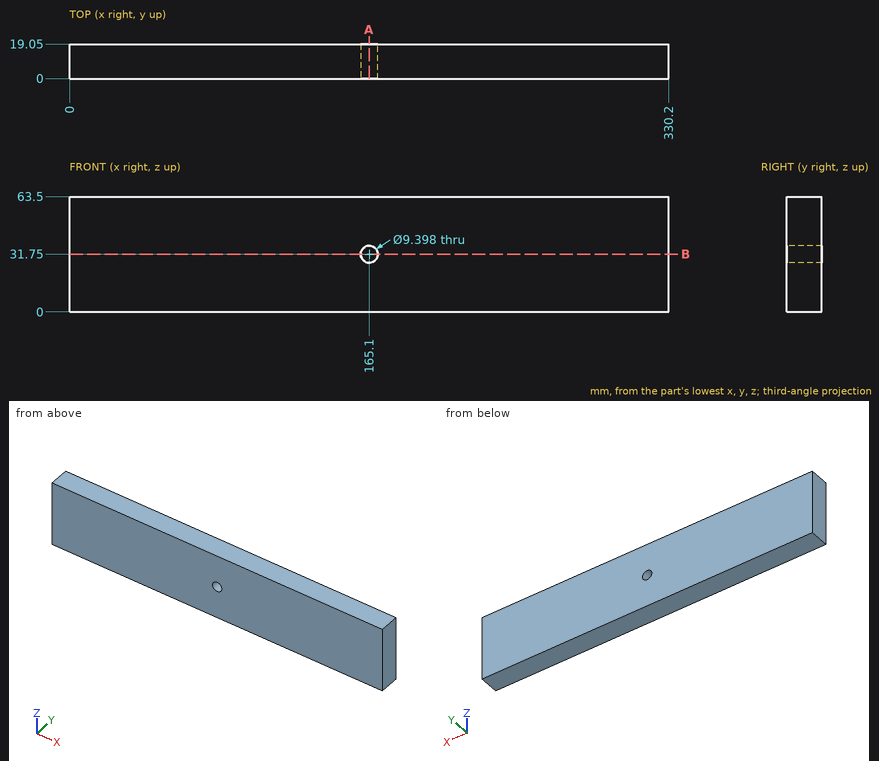
For this review, use the dimensioned drawing (mm, ordinates from the lowest corner) and the shaded views. Coordinates: 2 decimals unless noted, no trailing zeros. Loops run counter-clockwise (first coordinate to the right, second up) from the corner with the lowest first, then second, coordinate; pieces in that order, holes last. Notation, with made-up numbers: (89.25, 86.5) -> (99.25, 86.5) arc R11 ccw to (99.25, 100.5) -> close; hole circle Ø3 at (27, 43). An arc over 180 degrees is marked (long way). Use a Markdown table: item, result. Add a question column.
Item 1: We need section A-A, the plane x = 165.1. Write out the cut boundary in (y, z), and give its area (3 significant figures).
Item 2: Wall thickness on L1, parallel to X at y = 13.25, z = 31.75; L2, parallel to Z at x = 165.1, y = 14.75: over which ranges is each line inside the solid? List them lowest first. Write a range as from..to.
Item 3: We need section B-B, the plane z = 31.75. Write out the cut boundary in (x, y).
Numbers:
| question | item | result |
|---|---|---|
| 1 | outline | (0, 0) -> (19.05, 0) -> (19.05, 27.05) -> (0, 27.05) -> close; (0, 36.45) -> (19.05, 36.45) -> (19.05, 63.5) -> (0, 63.5) -> close |
| 1 | area | 1,030 mm^2 |
| 2 | L1 | x = 0..160.4, 169.8..330.2 |
| 2 | L2 | z = 0..27.05, 36.45..63.5 |
| 3 | outline | (0, 0) -> (160.4, 0) -> (160.4, 19.05) -> (0, 19.05) -> close; (169.8, 0) -> (330.2, 0) -> (330.2, 19.05) -> (169.8, 19.05) -> close |
